Can you work these out from the model? Positions are in its coordinate system, mm. A direction names the side the tool comes from. Coordinates: 2 decimals unless noted, no trailing zeros. Order: outer loops, then holes, each group sorted by start corner. A loop starts at its lowest first (then second) coordinate and runs counter-clockwise, first axis right, second up. Notation, with made-up numbers: (16, -19) -> (24, -19) arc R13 cw to (24, -15) -> close; hole circle Ø6 at (-37.75, -35). An arc over 180 degrees is marked (long way). Use a Markdown table: item, result. Add a question column.
1. We'd pull the mould along Y, two halves only. Please class faces 1 (the flat face through (-1, -63.5, 0)), 2 (the flat face through (1, -35, 9.525)), 3 (the flat face through (46, 25.4, 42)): pulls with the +Y half, pulls with the -Y half, needs draft (parallel to the pull), parting line crosses it, or undercut.
2. Suppose I cut it at C-C, the plane z = 1.5. List the corners of the cut face in (x, y) for me (3 decimals), then the cut area to 3 significant figures.
3. If I drill on line 1 along Y through (x, z) = (26.5, 29); line 2 along Z through (x, y) = (-26.5, -42) (3 decimals); line 3 along Y through (x, z) = (-0.5, 47), over which ranges is the centre line in solid material (lowest first)? Write a range as from..to.
4. For faces 4 (the flat face through (-4, -6.35, 30)), 5 (the cylindrical face through (45.8, -0.4, 38.1)), 6 (the flat face through (41.275, -1, 4)), 7 (the flat face through (46, -25.4, 42)), which set-ups out of +Z, -Z, +X, -X, +Y, -Y let a thin tool reach every point of the face, with its end or its side?
5. For pin 1 Ø2.5 at (y, z) = (-1, 40.5) entering from -X; pin 2 Ø1 at (y, z) = (-7, 51.5) entering from -X; pin 3 Ø22.5 at (x, y) = (67, 8) entering from -Z, each with a flat end and sliding along its axis, tell me the tip position at first contact or that it passes through.
6. Suppose I cut it at B-B, the plane y = 52. List the corners of the cut face in (x, z) for me (3 decimals), then the cut area to 3 significant figures.
7. Suppose I cut it at A-A, the plane x = 78. List the corners of the cut face in (y, z) for me (3 decimals).
```python
from build123d import *

# Parameters (mm, degrees)
F1_DEPTH = 63.5
F0_W     = 25.4
F0_H     = 19.05
F2_DEPTH = 25.4
F0_H_2   = 4.7498
F0_H_3   = 4.7752
F3_DEPTH = 6.35


with BuildPart() as f1:
    # F0 (on Front) → F1 (new body, symmetric)
    with BuildSketch(Plane.XZ):
        Polygon((22.225, 9.525), (-41.275, 9.525), (-41.275, -9.525), (41.275, -9.525), (41.275, 9.525), align=None)
    extrude(amount=F1_DEPTH, both=True)

    # F0 (on Front) → F2 (join, symmetric)
    with BuildSketch(Plane.XZ):
        with BuildLine():
            Line((22.225, 27.0002), (22.225, 9.525))
            Line((22.225, 9.525), (41.275, 9.525))
            Line((41.275, 9.525), (41.275, 27.0002))
            ThreePointArc((41.275, 27.0002), (45.9246798487, 38.2255201513), (57.15, 42.8752))
            Line((57.15, 42.8752), (59.9058770299, 42.8752))
            Line((59.9058770299, 42.8752), (59.9058770299, 61.9252))
            Line((59.9058770299, 61.9252), (57.15, 61.9252))
            add(Edge.make_bspline(
                [(53.9486358341, 61.7781656173), (55.0198111494, 61.8401017222), (56.0872015852, 61.8892118375), (57.15, 61.9252)],
                knots=[108.8616343251, 108.8616343251, 108.8616343251, 108.8616343251, 111.5045361635, 111.5045361635, 111.5045361635, 111.5045361635], degree=3))
            ThreePointArc((53.9486358341, 61.7781656173), (31.3472552962, 50.5368520719), (22.225, 27.0002))
        make_face()
        with Locations((72.6058770299, 52.4002)):
            Rectangle(F0_W, F0_H)
    extrude(amount=F2_DEPTH, both=True)

    # F0 (on Front) → F3 (join, symmetric)
    with BuildSketch(Plane.XZ):
        with BuildLine():
            add(Edge.make_bspline(
                [(-41.275, 9.525), (-40.7167454474, 34.9148619979), (9.8267188659, 59.2270055586), (53.9486358341, 61.7781656173)],
                knots=[0, 0, 0, 0, 108.8616343251, 108.8616343251, 108.8616343251, 108.8616343251], degree=3))
            Line((-41.275, 9.525), (22.225, 9.525))
            Line((22.225, 9.525), (22.225, 27.0002))
            ThreePointArc((22.225, 27.0002), (31.3472552962, 50.5368520719), (53.9486358341, 61.7781656173))
        make_face()
        Polygon((22.225, 9.525), (-41.275, 9.525), (-41.275, -9.525), (41.275, -9.525), (41.275, 9.525), align=None)
        with BuildLine():
            Line((22.225, 27.0002), (22.225, 9.525))
            Line((22.225, 9.525), (41.275, 9.525))
            Line((41.275, 9.525), (41.275, 27.0002))
            ThreePointArc((41.275, 27.0002), (45.9246798487, 38.2255201513), (57.15, 42.8752))
            Line((57.15, 42.8752), (59.9058770299, 42.8752))
            Line((59.9058770299, 42.8752), (59.9058770299, 61.9252))
            Line((59.9058770299, 61.9252), (57.15, 61.9252))
            add(Edge.make_bspline(
                [(53.9486358341, 61.7781656173), (55.0198111494, 61.8401017222), (56.0872015852, 61.8892118375), (57.15, 61.9252)],
                knots=[108.8616343251, 108.8616343251, 108.8616343251, 108.8616343251, 111.5045361635, 111.5045361635, 111.5045361635, 111.5045361635], degree=3))
            ThreePointArc((53.9486358341, 61.7781656173), (31.3472552962, 50.5368520719), (22.225, 27.0002))
        make_face()
        with BuildLine():
            ThreePointArc((57.15, 61.9252), (55.5476305332, 61.8884220397), (53.9486358341, 61.7781656173))
            add(Edge.make_bspline(
                [(53.9486358341, 61.7781656173), (55.0198111494, 61.8401017222), (56.0872015852, 61.8892118375), (57.15, 61.9252)],
                knots=[108.8616343251, 108.8616343251, 108.8616343251, 108.8616343251, 111.5045361635, 111.5045361635, 111.5045361635, 111.5045361635], degree=3))
        make_face()
        with Locations((72.6058770299, 52.4002)):
            Rectangle(F0_W, F0_H)
        with Locations((72.6058770299, 64.3001)):
            Rectangle(F0_W, F0_H_2)
        with Locations((72.6058770299, 40.4876)):
            Rectangle(F0_W, F0_H_3)
        Polygon((85.3058770299, 66.675), (85.3058770299, 61.9252), (85.3058770299, 42.8752), (85.3058770299, 38.1), (110.7058770299, 38.1), (110.7058770299, 66.675), align=None)
    extrude(amount=F3_DEPTH, both=True)

    # F0 (on Front) → F4 (revolve)
    with BuildSketch(Plane.XZ):
        Polygon((85.3058770299, 66.675), (85.3058770299, 61.9252), (85.3058770299, 42.8752), (85.3058770299, 38.1), (110.7058770299, 38.1), (110.7058770299, 66.675), align=None)
    revolve(axis=Axis((85.3058770299, 0, 52.3875), (0, 0, 1)))


solid = f1.part
```
Worked out:
| question | item | result |
|---|---|---|
| 1 | face 1 | pulls with the -Y half |
| 1 | face 2 | needs draft |
| 1 | face 3 | pulls with the +Y half |
| 2 | outline | (-41.275, -63.5) -> (41.275, -63.5) -> (41.275, 63.5) -> (-41.275, 63.5) -> close |
| 2 | area | 10,500 mm² |
| 3 | line 1 | y = -25.4..25.4 |
| 3 | line 2 | z = -9.525..9.525 |
| 3 | line 3 | y = -6.35..6.35 |
| 4 | face 4 | +Z, -X, -Y |
| 4 | face 5 | -Z, +Y, -Y |
| 4 | face 6 | -Z, +X, +Y, -Y |
| 4 | face 7 | +Z, +X, -X, -Y |
| 5 | pin 1 | stops at x = -18.55 |
| 5 | pin 2 | stops at x = 31.78 |
| 5 | pin 3 | stops at z = 38.1 |
| 6 | outline | (-41.275, -9.525) -> (41.275, -9.525) -> (41.275, 9.525) -> (-41.275, 9.525) -> close |
| 6 | area | 1,570 mm² |
| 7 | outline | (-25.4, 42.875) -> (-24.327, 42.875) -> (-24.327, 38.1) -> (24.327, 38.1) -> (24.327, 42.875) -> (25.4, 42.875) -> (25.4, 61.925) -> (24.327, 61.925) -> (24.327, 66.675) -> (-24.327, 66.675) -> (-24.327, 61.925) -> (-25.4, 61.925) -> close |
